Part model, mm, in its own coordinate system. Round coordinates to 2 decimals unless told otherwise and drop trailing zeros. Write each loop counter-clockwise with the first axis right and the second up, starting at its lowest first coordinate (ties: lowest second). Pieces come first, ordered by that corner, then holes. Notation, with made-up numbers: M 75.25,-6.75 L 110.25,-6.75 A22 cw 110.25,31.25 Z; hole C 3,-22 d4. An arc over 180 degrees is marked long. Use one line per item in the form item = value. Start each with the question number.
Item 1: Cut at A-A, the plane y = 18. Give the cut face in (x, z).
Item 2: Cut at C-C, the plane z = 2.4. State how many separate pieces and enclosed holes the cut face has, then the cut area to 3 significant figures.
Item 3: Flat gauge pins, fed straight in: pin 1 Ø5.5 at (x, y) = (46.5, -50) entering from -Z; pin 2 Ø3 at (x, y) = (18, 17) entering from +Z. Where does each tip first touch, or does it go through?
Item 4: Cut at B-B, the plane x = -46.5. Give the cut face in (y, z), then the cut area to 3 significant figures.
Item 5: Cut at D-D, the plane y = 50. Give the cut face in (x, z).
Item 6: Probe L1, parallel to Y at x = 18, z = 2.7; L2, parallel to Y at x = -46.5, z = 2.8; L3, parallel to X at y = 16.5, z = 0.4. List the from-to ranges inside material, lowest first.
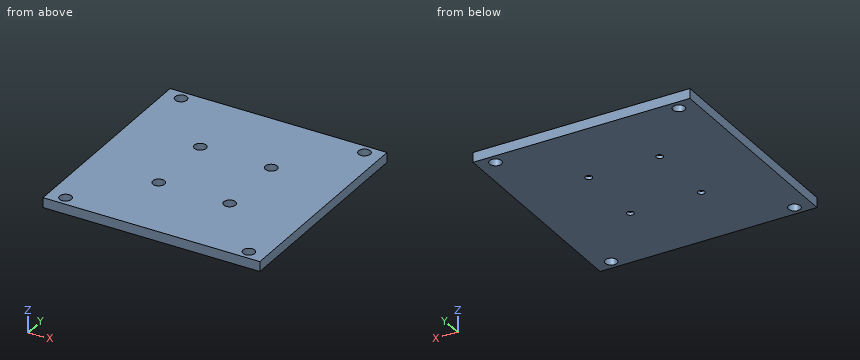
from build123d import *

# Parameters (mm, degrees)
F0_W     = 110
F0_H     = 110
F0_R     = 3
F1_DEPTH = 5
F2_R     = 1.75
F3_DEPTH = 5.001
F4_R     = 3
F5_DEPTH = 3.5


with BuildPart() as f1:
    # F0 (on Top) → F1 (new body)
    with BuildSketch(Plane.XY):
        Rectangle(F0_W, F0_H)
        with Locations((-46.5, -50)):
            Circle(F0_R, mode=Mode.SUBTRACT)
        with Locations((46.5, -50)):
            Circle(F0_R, mode=Mode.SUBTRACT)
        with Locations((-46.5, 50)):
            Circle(F0_R, mode=Mode.SUBTRACT)
        with Locations((46.5, 50)):
            Circle(F0_R, mode=Mode.SUBTRACT)
    extrude(amount=F1_DEPTH)

    # F2 (on face) → F3 (cut, through all)
    with BuildSketch(Plane.XY.offset(5)):
        with Locations((-18, 18)):
            Circle(F2_R)
        with Locations((18, 18)):
            Circle(F2_R)
        with Locations((-18, -18)):
            Circle(F2_R)
        with Locations((18, -18)):
            Circle(F2_R)
    extrude(amount=-F3_DEPTH, mode=Mode.SUBTRACT)

    # F4 (on face) → F5 (cut)
    with BuildSketch(Plane.XY.offset(5)):
        with Locations((-18, 18)):
            Circle(F4_R)
        with Locations((-18, -18)):
            Circle(F4_R)
        with Locations((18, 18)):
            Circle(F4_R)
        with Locations((18, -18)):
            Circle(F4_R)
    extrude(amount=-F5_DEPTH, mode=Mode.SUBTRACT)


solid = f1.part
Model answer:
q1.outline = M -55,0 L -19.75,0 L -19.75,1.5 L -21,1.5 L -21,5 L -55,5 Z; M -16.25,0 L 16.25,0 L 16.25,1.5 L 15,1.5 L 15,5 L -15,5 L -15,1.5 L -16.25,1.5 Z; M 19.75,0 L 55,0 L 55,5 L 21,5 L 21,1.5 L 19.75,1.5 Z
q2.separate_pieces = 1
q2.enclosed_holes = 8
q2.area = 11,900 mm²
q3.pin_1 = through
q3.pin_2 = 1.5
q4.outline = M -55,0 L -53,0 L -53,5 L -55,5 Z; M -47,0 L 47,0 L 47,5 L -47,5 Z; M 53,0 L 55,0 L 55,5 L 53,5 Z
q4.area = 490 mm²
q5.outline = M -55,0 L -49.5,0 L -49.5,5 L -55,5 Z; M -43.5,0 L 43.5,0 L 43.5,5 L -43.5,5 Z; M 49.5,0 L 55,0 L 55,5 L 49.5,5 Z
q6.L1 = -55 to -21, -15 to 15, 21 to 55
q6.L2 = -55 to -53, -47 to 47, 53 to 55
q6.L3 = -55 to -18.9, -17.1 to 17.1, 18.9 to 55
